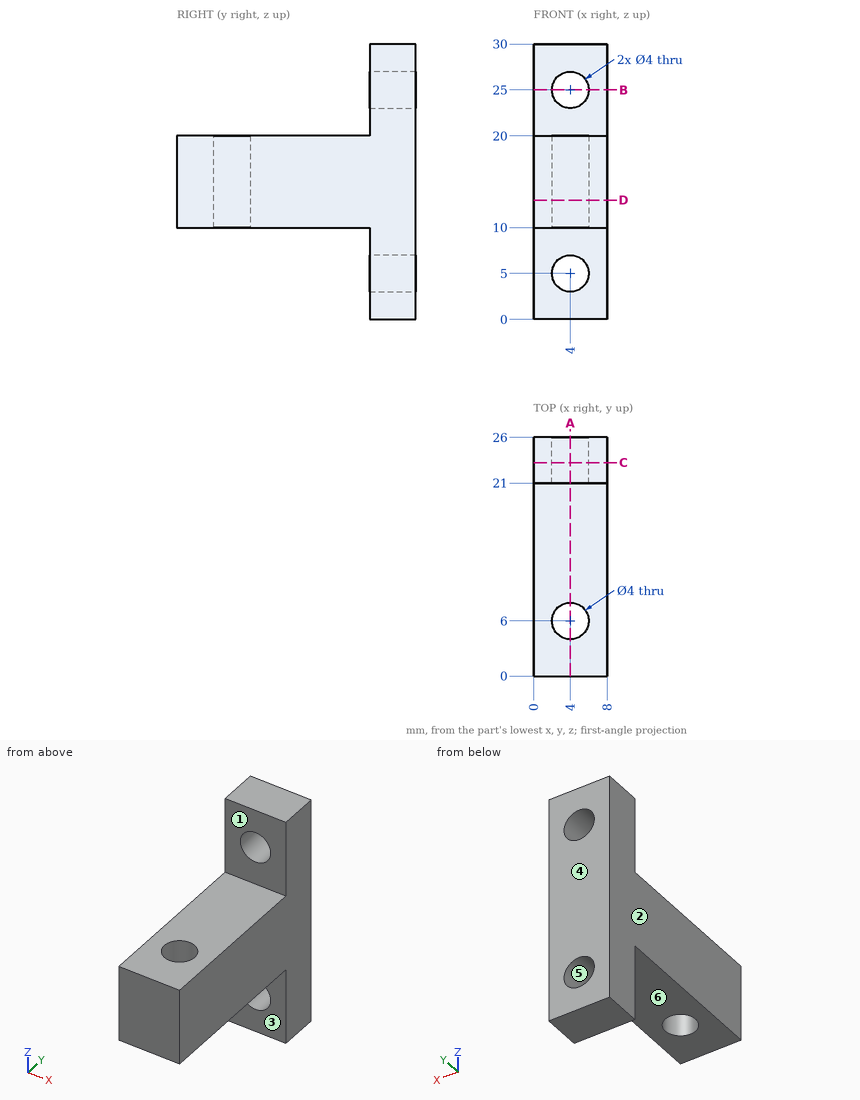
Design review of the part shown in the three views and the two pictorial views. Dimensions are in mm from the part's minimum x, y and z. A direction names the side the tool comes from. Round coordinates to 2 decimals unless told otherwise and drop trailing zeros. Order: outer loops, then holes, each group sorted by start corner. A loop starts at its lowest first (then second) coordinate and runs counter-clockwise, first axis right, second up. Notation, with made-up numbers: (26, 66) - (64, 66) arc R27 ccw to (64, 84) - close; hole circle Ø7 at (36, 33). An arc over 180 degrees is marked (long way). Answer in a Markdown table with one row per item.
(1) Take a section at B-B on z = 25. Write out the cut boundary in (x, y).
Result set:
| item | result |
|---|---|
| outline | (0, 21) - (2, 21) - (2, 26) - (0, 26) - close; (6, 21) - (8, 21) - (8, 26) - (6, 26) - close |
(2) For line 1 (X direction, y = 6, z = 17.25); line 2 (Y direction, x = 4, z = 12.5); line 3 (Z direction, x = 5, y = 15.25), list the stretches that pass through material, from the lowest coordinate up. Write a range as from..to.
Result set:
| item | result |
|---|---|
| line 1 | x = 0..2, 6..8 |
| line 2 | y = 0..4, 8..26 |
| line 3 | z = 10..20 |
(3) Clearance check with flat-ended pins moving along their axes: P1, Ø3, axis at x = 4, y = 6, coming from the +Z side; P2, Ø2, axis at x = 3, y = 18.5, coming from the +Z side; P3, Ø4, axis at x = 2, z = 24.5, coming from the -Y side; P4, Ø4, axis at x = 4.5, y = 10.5, coming from the -Z side. State where each tip first meets the part, or that it passes through.
Result set:
| item | result |
|---|---|
| P1 | passes through |
| P2 | stops at z = 20 |
| P3 | stops at y = 21 |
| P4 | stops at z = 10 |
(4) Take a section at A-A on x = 4. Write out the cut boundary in (y, z).
Result set:
| item | result |
|---|---|
| outline | (0, 10) - (4, 10) - (4, 20) - (0, 20) - close; (8, 10) - (21, 10) - (21, 7) - (26, 7) - (26, 23) - (21, 23) - (21, 20) - (8, 20) - close; (21, 0) - (26, 0) - (26, 3) - (21, 3) - close; (21, 27) - (26, 27) - (26, 30) - (21, 30) - close |
(5) Mouldability with a two-part tool opening along Z and no side actions: class the marked faces 4, 5 and 6 as released by +Z, released by -Z, zero draft, split by the parting line, or undercut.
Result set:
| item | result |
|---|---|
| face 4 | zero draft |
| face 5 | undercut |
| face 6 | released by -Z |
(6) Machinability: for the marked faces 1, 2 and 3, which of the approach directions +Z, -Z, +X, -X, +Y, -Y give a long, thin tool a straight path to every point of the face, cutting with its end or side? Answer none if there is none.
Result set:
| item | result |
|---|---|
| face 1 | +Z, +X, -X, -Y |
| face 2 | +Z, -Z, -X, +Y, -Y |
| face 3 | -Z, +X, -X, -Y |
(7) Take a section at C-C on y = 23.25. Write out the cut boundary in (x, z).
Result set:
| item | result |
|---|---|
| outline | (0, 0) - (8, 0) - (8, 30) - (0, 30) - close; hole circle Ø4 at (4, 5); hole circle Ø4 at (4, 25) |
(8) Take a section at D-D on z = 13. Write out the cut boundary in (x, y).
Result set:
| item | result |
|---|---|
| outline | (0, 0) - (8, 0) - (8, 26) - (0, 26) - close; hole circle Ø4 at (4, 6) |
